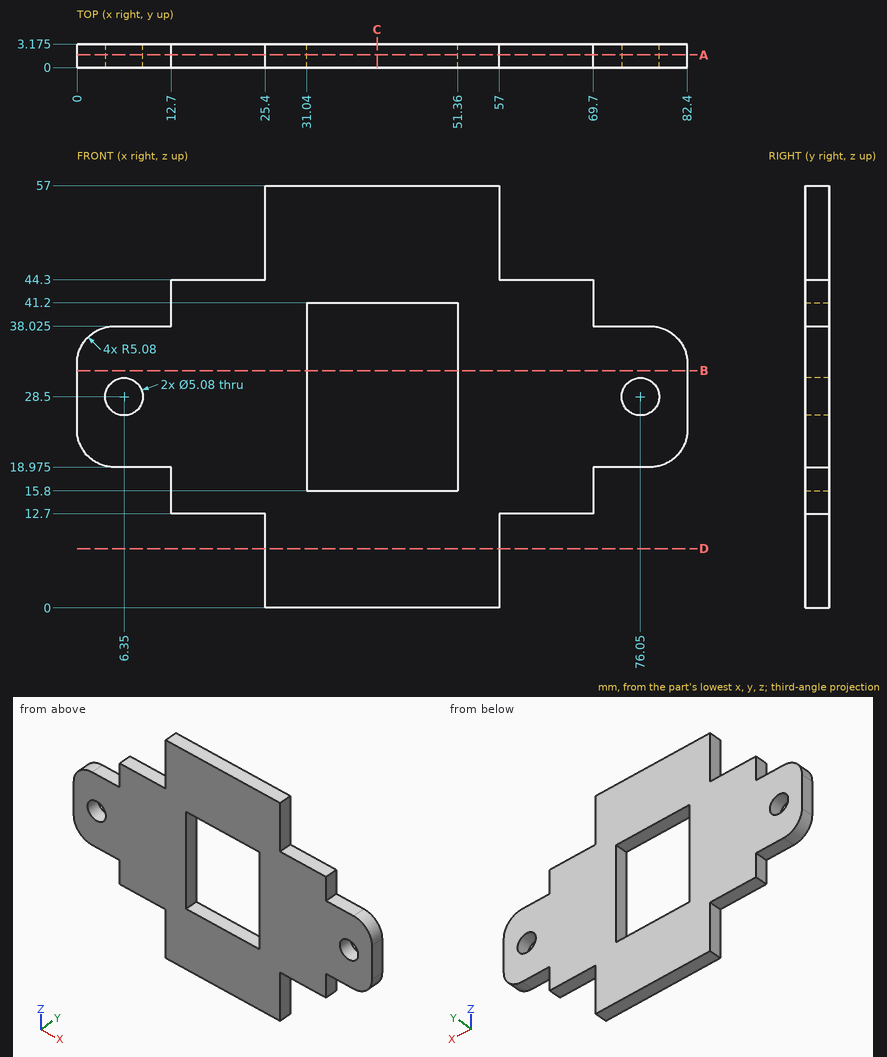
Verification items for this drawing (mm, ordinates from the low corner). Coordinates: 2 decimals unless noted, no trailing zeros. Order: outer loops, then holes, each group sorted by start corner. A loop starts at its lowest first (then second) coordinate and runs counter-clockwise, first axis right, second up. Notation, with made-up numbers: (24, 49) - (53, 49) arc R26 ccw to (53, 76) - close; hole circle Ø3 at (-10.75, 15). An arc over 180 degrees is marked (long way). Use one line per item in the form item = value.
1. Gauge pin test, flat ends, axial feed: pin 1 (1 mm diameter, centred on y = 2, z = 26.5, fed in from -X); pin 2 (1.6 mm diameter, centred on x = 20.5, y = 2, fed in from -Z); pin 3 (1.6 mm diameter, centred on x = 71.5, y = 1.5, fed in from -Z) (3 decimals); pin 4 (1.6 mm diameter, centred on x = 9, y = 2.5, fed in from +Z) (3 decimals). Record the tip position at first contact, or that the pin passes through.
Here are the results:
pin_1 = 0
pin_2 = 12.7
pin_3 = 18.975
pin_4 = 38.025
2. Section check A-A (y = 1.7). State how many separate pieces and enclosed holes the cut face has, then the cut area to 3 significant figures.
Here are the results:
separate_pieces = 1
enclosed_holes = 3
area = 2,510 mm²
3. Scan lines: line 1 (X direction, y = 2.7, z = 41); line 2 (X direction, y = 2.2, z = 28.5); line 3 (Z direction, x = 36.5, y = 0.6). Record each from-to range of solid material in increasing order.
Here are the results:
line_1 = 12.7 to 31.04, 51.36 to 69.7
line_2 = 0 to 3.81, 8.89 to 31.04, 51.36 to 73.51, 78.59 to 82.4
line_3 = 0 to 15.8, 41.2 to 57
4. Section check D-D (z = 8). Record the boundary of the cut face in (x, y) (3 decimals).
Here are the results:
outline = (25.4, 0) - (57, 0) - (57, 3.175) - (25.4, 3.175) - close
5. Section check C-C (x = 40.5). Record the boundary of the cut face in (y, z) (3 decimals).
Here are the results:
outline = (0, 0) - (3.175, 0) - (3.175, 15.8) - (0, 15.8) - close; (0, 41.2) - (3.175, 41.2) - (3.175, 57) - (0, 57) - close
6. Section check B-B (z = 32). Record the boundary of the cut face in (x, y) (3 decimals), then the cut area to 3 significant figures.
Here are the results:
outline = (0, 0) - (31.04, 0) - (31.04, 3.175) - (0, 3.175) - close; (51.36, 0) - (82.4, 0) - (82.4, 3.175) - (51.36, 3.175) - close
area = 197 mm²
